Source: CAD feature listing. Evaluate the final solid. Frame: model axes, mm. Round coordinates to 2 decimals unless told otherwise and drop trailing zeros. Loops run counter-clockwise (first coordinate to the right, second up) from the corner with the lowest first, then second, coordinate; pieces in that order, holes last. Notation, with made-up numbers: (72.5, 35) - (123.5, 35) arc R31 ccw to (123.5, 73) - close; hole circle Ø1 at (19, -14). An arc over 180 degrees is marked (long way). One line per question, with ' | ' between items.
from build123d import *

# Parameters (mm, degrees)
SKETCH1_W           = 40
SKETCH1_H           = 40
BOSS_EXTRUDE1_DEPTH = 60
SKETCH2_R           = 10
CUT_EXTRUDE1_DEPTH  = 40


with BuildPart() as part:
    # Sketch1 → Boss-Extrude1 (new body)
    with BuildSketch(Plane(origin=(0, 0, 0), x_dir=(1, 0, 0), z_dir=(0, 1, 0))):
        Rectangle(SKETCH1_W, SKETCH1_H)
    extrude(amount=BOSS_EXTRUDE1_DEPTH)

    # Sketch2 → Cut-Extrude1 (cut)
    with BuildSketch(Plane.ZY.offset(20)):
        with Locations((0, 40)):
            Circle(SKETCH2_R)
    extrude(amount=-CUT_EXTRUDE1_DEPTH, mode=Mode.SUBTRACT)


solid = part.part
1. Section query A-A, the plane y = 32. Return loops of the section in (x, z), plus the area to 3 significant figures.
Worked out:
outline: (-20, -20) - (20, -20) - (20, -6) - (-20, -6) - close; (-20, 6) - (20, 6) - (20, 20) - (-20, 20) - close | area: 1,120 mm2
2. Section query B-B, the plane x = -10. Return loops of the section in (y, z), plus the area to 3 significant figures.
Worked out:
outline: (0, -20) - (60, -20) - (60, 20) - (0, 20) - close; hole circle Ø20 at (40, 0) | area: 2,090 mm2
3. Section query C-C, the plane z = 0. Return loops of the section in (x, y).
Worked out:
outline: (-20, 0) - (20, 0) - (20, 30) - (-20, 30) - close; (-20, 50) - (20, 50) - (20, 60) - (-20, 60) - close
4. Material intervals for probe 1 along Y at (x, z) = (2, 0); probe 2 along Y at (x, z) = (5.5, 3); probe 3 along Z at (x, y) = (-15, 43), sorted ascending.
Worked out:
probe 1: y = 0 to 30, 50 to 60 | probe 2: y = 0 to 30.46, 49.54 to 60 | probe 3: z = -20 to -9.54, 9.54 to 20
5. Mould query, pull axis Y, two halves, no side actions, for faces 1 (the flat face through (0, 60, 0)), 2 (the flat face through (20, 29.6, 0.3)), 3 (the cylindrical face through (-0.28, 30.24, -2.17)). Classes: released by +Y, released by -Y, zero draft, split by the parting line, or undercut.
Worked out:
face 1: released by +Y | face 2: zero draft | face 3: undercut
6. Contact query for a flat-ended pin moving along its axis: P1, Ø12, axis at y = 42.5, z = -3.5, coming from the +X side. Output: stop coordinate, or through.
Worked out:
P1: stops at x = 20
